Could you check a few things on this model? Use its own coordinates, in mm. A direction names the side the tool comes from. Round coordinates to 2 decimals unless told otherwise and drop trailing zeros. Loops run counter-clockwise (first coordinate to the right, second up) from the corner with the lowest first, then second, coordinate; pieces in that order, holes last. Notation, with made-up numbers: M 34,14.25 L 68,14.25 A19 ccw 68,28.25 Z; hole C 42,-25 d4. An arc over 180 degrees is marked long. Answer in a Markdown table with one row per item.
```python
from build123d import *

# Parameters (mm, degrees)
SKETCH1_R             = 1.7
BOSS_EXTRUDE1_DEPTH   = 5
BOSS_EXTRUDE1_2_DEPTH = 5
BOSS_EXTRUDE2_DEPTH   = 12.55
BOSS_EXTRUDE3_DEPTH   = 5


with BuildPart() as part:
    # Sketch1 → Boss-Extrude1 (new body)
    with BuildSketch(Plane.XY):
        with BuildLine():
            Line((3.688712639, 26.875410947), (13.823430903, 15.8))
            Line((13.823430903, 15.8), (-13.823430903, 15.8))
            Line((-13.823430903, 15.8), (-3.688712639, 26.875410947))
            ThreePointArc((-3.688712639, 26.875410947), (0, 28.5), (3.688712639, 26.875410947))
        make_face()
        with Locations((0, 23.5)):
            Circle(SKETCH1_R, mode=Mode.SUBTRACT)
    extrude(amount=BOSS_EXTRUDE1_DEPTH)



with BuildPart() as body_2:
    # Sketch1 → Boss-Extrude1 2 (new body)
    with BuildSketch(Plane.XY):
        with BuildLine():
            ThreePointArc((3.688712639, -26.875410947), (0, -28.5), (-3.688712639, -26.875410947))
            Line((-3.688712639, -26.875410947), (-13.823430903, -15.8))
            Line((-13.823430903, -15.8), (13.823430903, -15.8))
            Line((13.823430903, -15.8), (3.688712639, -26.875410947))
        make_face()
        with Locations((0, -23.5)):
            Circle(SKETCH1_R, mode=Mode.SUBTRACT)
    extrude(amount=BOSS_EXTRUDE1_2_DEPTH)


with BuildPart() as part_1:
    add(part.part)

    add(body_2.part)  # Boss-Extrude2 merges body 2
    # Sketch2 → Boss-Extrude2 (add)
    with BuildSketch(Plane.XY.offset(5)):
        Polygon((-13.823430903, -15.8), (13.823430903, -15.8), (9.52262653, -20.5), (-9.52262653, -20.5), align=None)
        Polygon((-9.52262653, 20.5), (-13.823430903, 15.8), (13.823430903, 15.8), (9.52262653, 20.5), align=None)
    extrude(amount=BOSS_EXTRUDE2_DEPTH)

    # Sketch3 → Boss-Extrude3 (add)
    with BuildSketch(Plane.XY.offset(17.55)):
        with BuildLine():
            Line((-13.823430903, 15.8), (-13.823430903, -15.8))
            Line((-13.823430903, -15.8), (-9.52262653, -20.5))
            Line((-9.52262653, -20.5), (9.52262653, -20.5))
            Line((9.52262653, -20.5), (13.823430905, -15.8))
            ThreePointArc((13.823430905, -15.8), (2.711210982, -1e-09), (13.823430903, 15.8))
            Line((13.823430903, 15.8), (9.52262653, 20.5))
            Line((9.52262653, 20.5), (-9.52262653, 20.5))
            Line((-9.52262653, 20.5), (-13.823430903, 15.8))
        make_face()
    extrude(amount=BOSS_EXTRUDE3_DEPTH)


solid = part_1.part
```
1) If we mould it in two halves opening along Y, with no side actions, what happens to faces 5 (the face through (0, 20.5, 14)), 6 (the face through (-2, -24, 5)), 7 (the face through (-0.221, 25.186, 2.465))? For each: released by +Y, released by -Y, zero draft, split by the parting line, or undercut.
Computed:
| item | result |
|---|---|
| face 5 | released by +Y |
| face 6 | zero draft |
| face 7 | undercut |
2) I need wall thicknesses on line 1 (Y direction, x = -8, z = 9.5); line 2 (Z direction, x = -7, y = -4); line 3 (Y direction, x = -10.75, z = 9.25). Which ranges of each line are inside material? Lowest first, please.
Computed:
| item | result |
|---|---|
| line 1 | y = -20.5 to -15.8, 15.8 to 20.5 |
| line 2 | z = 17.55 to 22.55 |
| line 3 | y = -19.16 to -15.8, 15.8 to 19.16 |
3) Which directions (+Z, -Z, +X, -X, +Y, -Y) give clear straight access to the entire face, cutting with the end or side of a thin tool? Please do faces 1 (the face through (-0.1, 28.5, 2.5)), 2 (the face through (-3, 0, 17.55)), 3 (the face through (0, -20.5, 14)), 4 (the face through (0.1, 25.4, 5)).
Computed:
| item | result |
|---|---|
| face 1 | +Z, -Z, +Y |
| face 2 | -Z, +X, -X |
| face 3 | +Z, +X, -X, -Y |
| face 4 | +Z, +X, -X, +Y |
4) I want a section at B-B, the plane x = 0. Please give me the cut outline in (y, z).
Computed:
| item | result |
|---|---|
| outline | M -28.5,0 L -25.2,0 L -25.2,5 L -28.5,5 Z; M -21.8,0 L -15.8,0 L -15.8,17.55 L 15.8,17.55 L 15.8,0 L 21.8,0 L 21.8,5 L 20.5,5 L 20.5,22.55 L -20.5,22.55 L -20.5,5 L -21.8,5 Z; M 25.2,0 L 28.5,0 L 28.5,5 L 25.2,5 Z |
5) I want a section at C-C, the plane z = 16. Please give me the cut outline in (x, y), plus the area to 3 significant figures.
Computed:
| item | result |
|---|---|
| outline | M -13.82,-15.8 L -9.52,-20.5 L 9.52,-20.5 L 13.82,-15.8 Z; M -13.82,15.8 L 13.82,15.8 L 9.52,20.5 L -9.52,20.5 Z |
| area | 219 mm² |
6) I want a section at D-D, the plane y = 23.5. Please give me the cut outline in (x, z).
Computed:
| item | result |
|---|---|
| outline | M -6.78,0 L -1.7,0 L -1.7,5 L -6.78,5 Z; M 1.7,0 L 6.78,0 L 6.78,5 L 1.7,5 Z |
7) Will these pins go through, and if not, where does the flat tip stop? P1, Ø9, axis at x = -4.5, z = 15, coming from the -Y side; P2, Ø6, axis at x = -5, y = -12, coming from the -Z side; P3, Ø4, axis at x = -1, y = -24.5, coming from the +Z side.
Computed:
| item | result |
|---|---|
| P1 | stops at y = -20.5 |
| P2 | stops at z = 17.55 |
| P3 | stops at z = 5 |
8) I want a section at A-A, the plane z = 3.75. Please give me the cut outline in (x, y).
Computed:
| item | result |
|---|---|
| outline | M -13.82,-15.8 L -3.69,-26.88 A5 ccw 3.69,-26.88 L 13.82,-15.8 Z; M -13.82,15.8 L 13.82,15.8 L 3.69,26.88 A5 ccw -3.69,26.88 Z; hole C 0,-23.5 d3.4; hole C 0,23.5 d3.4 |
